Autodesk Inventor part; units mm, degrees
ref_plane "YZ Plane" through (0, 0, 0) normal (1, 0, 0) x (0, 1, 0)
ref_plane "XZ Plane" through (0, 0, 0) normal (0, 1, 0) x (-1, 0, 0)
ref_plane "XY Plane" through (0, 0, 0) normal (0, 0, 1) x (1, 0, 0)
sketch "Boceto1" plane through (0, 0, 0) normal (0, 1, 0) x (-1, 0, 0)
  line L0 (0, 0) -> (50, 0)
  line L1 (50, 0) -> (50, -15)
  line L2 (50, -15) -> (0, -15)
  line L3 (0, -15) -> (0, 0)
  dimension "d0" = 50
  dimension "d1" = 15
extrude "Extrusión1" add sketch "Boceto1" along normal blind 10
sketch "Boceto2" plane through (0, 10, 0) normal (0, 1, 0) x (1, 0, 0)
  line L0 (-50, 15) -> (-50, 0)
  line L1 (-50, 0) -> (0, 0)
  point P0 (-42.5, 7.5)
  dimension "d4" = 7.5
  dimension "d12" = 7.5
hole "Agujero1" at (-42.5, 10, -7.5) direction (0, -1, 0) diameter 5.2 end through all counterbore diameter 11.7 counterbore depth 4
sketch "Boceto3" plane through (0, 0, 0) normal (1, 0, 0) x (0, 0, -1)
  point P0 (0, 0)
chamfer "Chaflán1" distance 20 distance2 10 1 edges at (0, 10, -7.5) measured on face at (-12.2309, 10, -7.265)
sketch "Boceto4" plane through (0, 0, 0) normal (0, -1, 0) x (1, 0, 0)
  line L0 (0, -15) -> (-50, -15)
  line L1 (0, -15) -> (-50, -15)
  line L2 (-50, -15) -> (-50, 0)
  line L3 (-50, 0) -> (0, 0)
  line L4 (0, 0) -> (0, -15)
extrude "Extrusión2" add sketch "Boceto4" along normal blind 2
sketch "Boceto5" plane through (-42.5, 0, -7.5) normal (0, 1, 0) x (1, 0, 0)
  circle A0 centre (0, 0) radius 2.6
  point P0 (42.5, -7.5)
hole "Agujero2" at (-42.5, 0, -7.5) direction (0, -1, 0) diameter 5.2 end through all
properties part number "cuña 5cm"
Geometry: final body of the model. Coordinates: model frame, mm. A direction names the side the tool comes from. Round coordinates to 2 decimals unless told otherwise and drop trailing zeros. Order: outer loops, then holes, each group sorted by start corner. A loop starts at its lowest first (then second) coordinate and runs counter-clockwise, first axis right, second up. Notation, with made-up numbers: (-0.75, 68.5) -> (7.25, 68.5) arc R27 cw to (7.25, 94.5) -> close; hole circle Ø6 at (67.5, 82.25). An arc over 180 degrees is marked (long way). Use one line per item in the form item = value. Start each with the question number.
1. Reachability of faces 4 (the face through (-50, 4, -8)), 5 (the face through (-36.79, 7.97, -8.77)) from +Z, -Z, +X, -X, +Y, -Y: full face, straight path, thin tool, end or side. Return the list, or none.
2. Draft query along X for faces 1 (the face through (-41, 6, -5)), 2 (the face through (-31, 10, -7)), 3 (the face through (-10, 5, -8)). Return one class per face: pulls with the +X half, pulls with the -X half, needs draft (parallel to the pull), parting line crosses it, or undercut.
3. Cut plane D-D (z = -3.75). Return the cut outline in (x, y).
4. Pin query (flat end, axial travel): pin 1 Ø2 at (x, y) = (-37, 7) entering from +Z; pin 2 Ø3.5 at (x, z) = (-40.5, -5.5) entering from +Y; pin 3 Ø3 at (y, z) = (7.5, -6) entering from +X. Return the tip coordinate at first contact, or that it passes through.
5. Cut plane A-A (x = -42.5). Return the cut outline in (y, z), then the cut area to 3 significant figures.
6. Cut plane C-C (y = -1). Return the cut outline in (x, z).
7. Line query: probe 1 along Z at (x, y) = (-42.5, 8.05); probe 2 along Z at (x, y) = (-42.5, 0.25); probe 3 along X at (y, z) = (2.25, -7.5). Output: solid intervals per line, ascending.
8. Cut plane B-B (z = -7.5). Return the cut outline in (x, y), then the cut area to 3 significant figures.
Solution:
q1.face_4 = +Z, -Z, -X, +Y, -Y
q1.face_5 = +Y
q2.face_1 = undercut
q2.face_2 = needs draft
q2.face_3 = pulls with the +X half
q3.outline = (-50, -2) -> (0, -2) -> (0, 0) -> (-20, 10) -> (-38.01, 10) -> (-38.01, 6) -> (-46.99, 6) -> (-46.99, 10) -> (-50, 10) -> close
q4.pin_1 = 0
q4.pin_2 = 6
q4.pin_3 = -12
q5.outline = (-2, -15) -> (10, -15) -> (10, -13.35) -> (6, -13.35) -> (6, -10.1) -> (-2, -10.1) -> close; (-2, -4.9) -> (6, -4.9) -> (6, -1.65) -> (10, -1.65) -> (10, 0) -> (-2, 0) -> close
q5.area = 91.6 mm^2
q6.outline = (-50, -15) -> (0, -15) -> (0, 0) -> (-50, 0) -> close; hole circle Ø5.2 at (-42.5, -7.5)
q7.probe_1 = -15 to -13.35, -1.65 to 0
q7.probe_2 = -15 to -10.1, -4.9 to 0
q7.probe_3 = -50 to -45.1, -39.9 to -4.5
q8.outline = (-50, -2) -> (-45.1, -2) -> (-45.1, 6) -> (-48.35, 6) -> (-48.35, 10) -> (-50, 10) -> close; (-39.9, -2) -> (0, -2) -> (0, 0) -> (-20, 10) -> (-36.65, 10) -> (-36.65, 6) -> (-39.9, 6) -> close
q8.area = 412 mm^2
